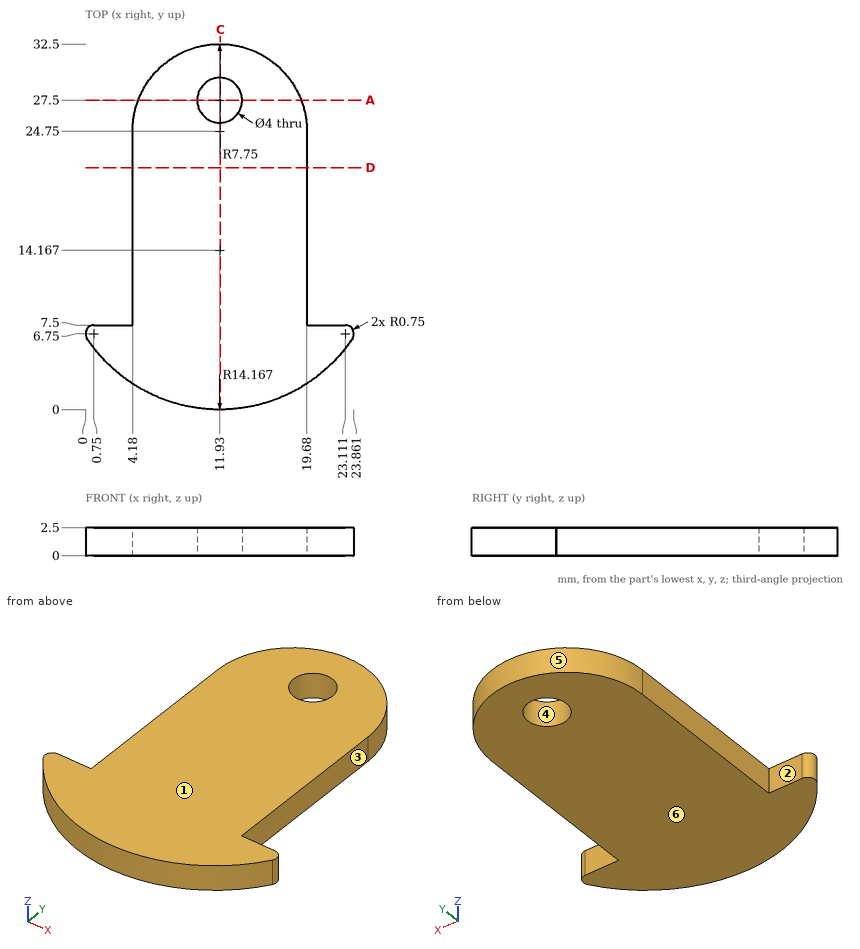
Geometry check sheet. Reference: drawing and pictorial views, mm from the part's lowest x, y, z. A direction names the side the tool comes from. Give positions to 0.01 mm unless a question says otherwise; leave off trailing zeros. Loops run counter-clockwise (first coordinate to the right, second up) from the corner with the lowest first, then second, coordinate; pieces in that order, holes last.
1. Mould release check, pull along Y, two halves, no side actions. Record for the marked faces 4, 5 and 6: released by +Y, released by -Y, zero draft, split by the parting line, or undercut.
2. Section check A-A, the plane y = 27.5. Enter the section's corners in (x, z) (1 decimal), then the cut area to 3 significant figures.
3. Set-up check for the marked faces 1, 2 and 3: record each of +Z, -Z, +X, -X, +Y, -Y from which the full face is reachable in a straight line by a thin tool's end or side.
4. Section check C-C, the plane x = 12. Enter the section's corners in (y, z).
5. Go/stop test with flat-tipped pins: pin 1 Ø0.8 at (y, z) = (18.5, 0.5) entering from -X; pin 2 Ø0.8 at (x, z) = (22, 1.5) entering from +Y; pin 3 Ø1.5 at (y, z) = (14.5, 2) entering from +X; pin 4 Ø2.5 at (x, y) = (11.93, 27.5) entering from -Z. Record where each tip stops, or that it passes through.
6. Section check D-D, the plane y = 21.5. Enter the section's corners in (x, z).
7. Thickness scan on line 1 (Y direction, x = 12, z = 2.25); line 2 (X direction, y = 14, z = 1.65); line 3 (Y direction, x = 10.5, z = 1.7) (1 decimal). Record the ranges inside material, lowest first.
Geometry says:
1. face 4: undercut
1. face 5: released by +Y
1. face 6: zero draft
2. outline: (4.7, 0) - (9.9, 0) - (9.9, 2.5) - (4.7, 2.5) - close; (13.9, 0) - (19.2, 0) - (19.2, 2.5) - (13.9, 2.5) - close
2. area: 26.2 mm2
3. face 1: +Z, +X, -X, +Y, -Y
3. face 2: +Z, -Z, -X, +Y
3. face 3: +Z, -Z, +X, +Y
4. outline: (0, 0) - (25.5, 0) - (25.5, 2.5) - (0, 2.5) - close; (29.5, 0) - (32.5, 0) - (32.5, 2.5) - (29.5, 2.5) - close
5. pin 1: stops at x = 4.18
5. pin 2: stops at y = 7.5
5. pin 3: stops at x = 19.68
5. pin 4: passes through
6. outline: (4.18, 0) - (19.68, 0) - (19.68, 2.5) - (4.18, 2.5) - close
7. line 1: y = 0 to 25.5, 29.5 to 32.5
7. line 2: x = 4.18 to 19.68
7. line 3: y = 0.1 to 26.1, 28.9 to 32.4
